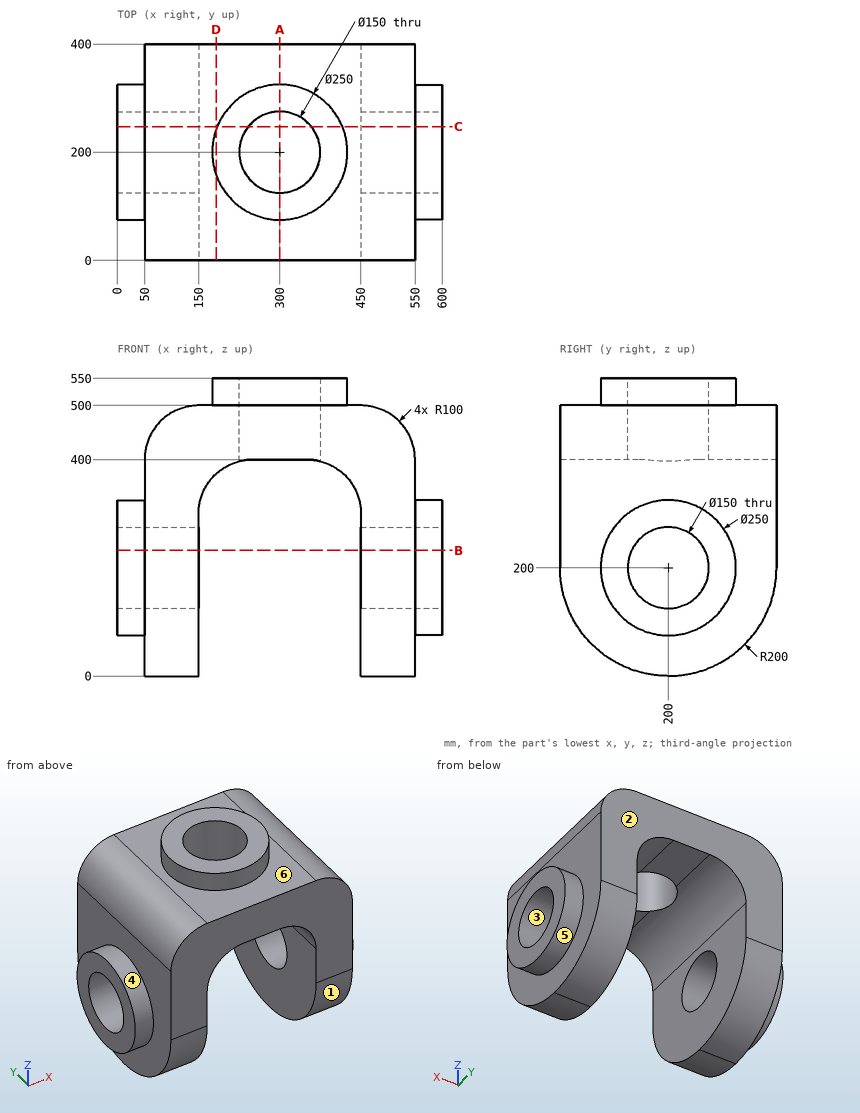
Here's the drawing with two shaded views (mm, measured from the low corner). I have some questions. A direction names the side the tool comes from. Coordinates: 2 decimals unless noted, no trailing zeros. Loops run counter-clockwise (first coordinate to the right, second up) from the corner with the lowest first, then second, coordinate; pieces in that order, holes last. Notation, with made-up numbers: (78.25, 34.25) -> (115.25, 34.25) arc R21 cw to (115.25, 43.25) -> close; hole circle Ø7 at (58.25, 84.25). An arc over 180 degrees is marked (long way). Answer as a JSON object with one key per item and string values.
1) For the marked faces 4, 5 and 6, which set-ups out of +Z, -Z, +X, -X, +Y, -Y let a thin tool reach every point of the face, with its end or its side?
Results:
{"face 4": "-X", "face 5": "+X", "face 6": "+Z"}
2) Thinking about a two-plate mould opening in Y: for the marked faces 1, 2 and 3, which applies, pulls with the +Y half, pulls with the -Y half, needs draft (parallel to the pull), parting line crosses it, or undercut?
Results:
{"face 1": "pulls with the -Y half", "face 2": "pulls with the +Y half", "face 3": "undercut"}
3) Imagine slicing it at D-D (x = 182.5). Please give me the cut outline in (y, z), then the cut area to 3 significant figures.
Results:
{"outline": "(0, 373.78) -> (400, 373.78) -> (400, 500) -> (242.65, 500) -> (242.65, 550) -> (157.35, 550) -> (157.35, 500) -> (0, 500) -> close", "area": "54,800 mm^2"}
4) For P1, Ø8, axis at y = 145.5, z = 349.5, coming from the +X side; P2, Ø4, axis at y = 109.5, z = 396, coming from the -X side; P3, Ø2, axis at y = 53, z = 427.5, coming from the -X side, each with a flat end and sliding along its axis, tell me the tip position at first contact or that it passes through.
Results:
{"P1": "stops at x = 550", "P2": "stops at x = 50", "P3": "stops at x = 53.58"}
5) Imagine slicing it at B-B (z = 232). Please give me the cut outline in (x, y).
Results:
{"outline": "(0, 79.17) -> (50, 79.17) -> (50, 0) -> (150, 0) -> (150, 132.17) -> (0, 132.17) -> close; (0, 267.83) -> (150, 267.83) -> (150, 400) -> (50, 400) -> (50, 320.83) -> (0, 320.83) -> close; (450, 0) -> (550, 0) -> (550, 79.17) -> (600, 79.17) -> (600, 132.17) -> (450, 132.17) -> close; (450, 267.83) -> (600, 267.83) -> (600, 320.83) -> (550, 320.83) -> (550, 400) -> (450, 400) -> close"}
6) Imagine slicing it at A-A (x = 300). Please give me the cut outline in (y, z).
Results:
{"outline": "(0, 400) -> (125, 400) -> (125, 550) -> (75, 550) -> (75, 500) -> (0, 500) -> close; (275, 400) -> (400, 400) -> (400, 500) -> (325, 500) -> (325, 550) -> (275, 550) -> close"}
7) If I drill on line 1 (Y direction, x = 300, z = 450); line 2 (X direction, y = 294.5, z = 101); line 3 (X direction, y = 237, z = 103), over which ranges is the centre line in solid material (lowest first)?
Results:
{"line 1": "y = 0 to 125, 275 to 400", "line 2": "x = 50 to 150, 450 to 550", "line 3": "x = 0 to 150, 450 to 600"}
8) Imagine slicing it at C-C (y = 247.5). Count the separate pieces of the cut face and the enclosed holes in it, then the cut area to 3 significant figures.
Results:
{"separate pieces": "4", "enclosed holes": "0", "area": "111,000 mm^2"}
